The model under review builds one solid part; all positions refer to its coordinate system, in mm. Coordinates: 2 decimals unless noted, no trailing zeros. Loops run counter-clockwise (first coordinate to the right, second up) from the corner with the lowest first, then second, coordinate; pieces in that order, holes last. Notation, with made-up numbers: M -16,79 L 31,79 A8 cw 31,91 Z; hole C 34,-31 d7. An arc over 180 degrees is marked long. One line per item, written item: value.
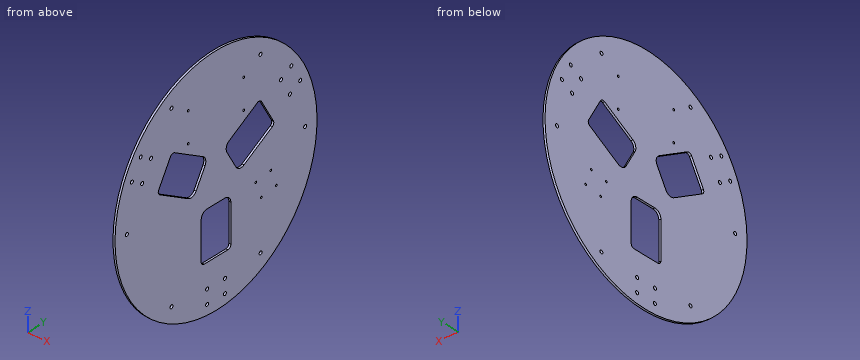
```python
from build123d import *

# Parameters (mm, degrees)
SKETCH_1_R      = 170
SKETCH_1_R_2    = 2.5
SKETCH_1_R_3    = 1.5
EXTRUDE_1_DEPTH = 3


with BuildPart() as part:
    # 草图1 → 凸台-拉伸1 (new body)
    with BuildSketch(Plane(origin=(0, 0, 0), x_dir=(0, 0, -1), z_dir=(1, 0, 0))):
        Circle(SKETCH_1_R)
        with Locations((155, 15)):
            Circle(SKETCH_1_R_2, mode=Mode.SUBTRACT)
        with Locations((135, 15)):
            Circle(SKETCH_1_R_2, mode=Mode.SUBTRACT)
        with Locations(Location((135, -15, 0), (0, 0, 180))):
            Circle(SKETCH_1_R_2, mode=Mode.SUBTRACT)
        with Locations(Location((155, -15, 0), (0, 0, 180))):
            Circle(SKETCH_1_R_2, mode=Mode.SUBTRACT)
        with Locations((-90.490381057, 126.733937587)):
            Circle(SKETCH_1_R_2, mode=Mode.SUBTRACT)
        with Locations((-80.490381057, 109.413429511)):
            Circle(SKETCH_1_R_2, mode=Mode.SUBTRACT)
        with Locations(Location((-54.509618943, 124.413429511, 0), (0, 0, 180))):
            Circle(SKETCH_1_R_2, mode=Mode.SUBTRACT)
        with Locations(Location((-64.509618943, 141.733937587, 0), (0, 0, 180))):
            Circle(SKETCH_1_R_2, mode=Mode.SUBTRACT)
        with Locations((-64.509618943, -141.733937587)):
            Circle(SKETCH_1_R_2, mode=Mode.SUBTRACT)
        with Locations((-54.509618943, -124.413429511)):
            Circle(SKETCH_1_R_2, mode=Mode.SUBTRACT)
        with Locations(Location((-80.490381057, -109.413429511, 0), (0, 0, 180))):
            Circle(SKETCH_1_R_2, mode=Mode.SUBTRACT)
        with Locations(Location((-90.490381057, -126.733937587, 0), (0, 0, 180))):
            Circle(SKETCH_1_R_2, mode=Mode.SUBTRACT)
        with Locations((-70, 46.6)):
            Circle(SKETCH_1_R_3, mode=Mode.SUBTRACT)
        with Locations((-113.2, 46.6)):
            Circle(SKETCH_1_R_3, mode=Mode.SUBTRACT)
        with Locations(Location((-113.2, -46.6, 0), (0, 0, 180))):
            Circle(SKETCH_1_R_3, mode=Mode.SUBTRACT)
        with Locations(Location((-70, -46.6, 0), (0, 0, 180))):
            Circle(SKETCH_1_R_3, mode=Mode.SUBTRACT)
        with Locations((0, -150)):
            Circle(SKETCH_1_R_2, mode=Mode.SUBTRACT)
        with Locations((-129.903810568, -75)):
            Circle(SKETCH_1_R_2, mode=Mode.SUBTRACT)
        with Locations((-129.903810568, 75)):
            Circle(SKETCH_1_R_2, mode=Mode.SUBTRACT)
        with Locations((0, 150)):
            Circle(SKETCH_1_R_2, mode=Mode.SUBTRACT)
        with Locations((129.903810568, 75)):
            Circle(SKETCH_1_R_2, mode=Mode.SUBTRACT)
        with Locations((129.903810568, -75)):
            Circle(SKETCH_1_R_2, mode=Mode.SUBTRACT)
        with Locations((54.035898385, 101.592921435)):
            Circle(SKETCH_1_R_3, mode=Mode.SUBTRACT)
        with Locations((34.035898385, 66.951905284)):
            Circle(SKETCH_1_R_3, mode=Mode.SUBTRACT)
        with Locations((57.892304845, 76.27241336)):
            Circle(SKETCH_1_R_3, mode=Mode.SUBTRACT)
        with Locations((30.179491924, 92.27241336)):
            Circle(SKETCH_1_R_3, mode=Mode.SUBTRACT)
        with BuildLine():
            Line((100, 0), (100, 20))
            ThreePointArc((100, 20), (98.535533906, 23.535533906), (95, 25))
            Line((95, 25), (40, 25))
            ThreePointArc((40, 25), (32.928932188, 22.071067812), (30, 15))
            Line((30, 15), (30, -15))
            ThreePointArc((30, -15), (32.928932188, -22.071067812), (40, -25))
            Line((40, -25), (95, -25))
            ThreePointArc((95, -25), (98.535533906, -23.535533906), (100, -20))
            Line((100, -20), (100, 0))
        make_face(mode=Mode.SUBTRACT)
        with BuildLine():
            Line((-50, 86.602540378), (-67.320508076, 76.602540378))
            ThreePointArc((-67.320508076, 76.602540378), (-69.650137207, 73.566508585), (-69.150635095, 69.77241336))
            Line((-69.150635095, 69.77241336), (-41.650635095, 22.141016151))
            ThreePointArc((-41.650635095, 22.141016151), (-35.578571508, 17.481757888), (-27.990381057, 18.480762114))
            Line((-27.990381057, 18.480762114), (-2.009618943, 33.480762114))
            ThreePointArc((-2.009618943, 33.480762114), (2.64963932, 39.5528257), (1.650635095, 47.141016151))
            Line((1.650635095, 47.141016151), (-25.849364905, 94.77241336))
            ThreePointArc((-25.849364905, 94.77241336), (-28.885396699, 97.102042491), (-32.679491924, 96.602540378))
            Line((-32.679491924, 96.602540378), (-50, 86.602540378))
        make_face(mode=Mode.SUBTRACT)
        with BuildLine():
            Line((-50, -86.602540378), (-32.679491924, -96.602540378))
            ThreePointArc((-32.679491924, -96.602540378), (-28.885396699, -97.102042491), (-25.849364905, -94.77241336))
            Line((-25.849364905, -94.77241336), (1.650635095, -47.141016151))
            ThreePointArc((1.650635095, -47.141016151), (2.64963932, -39.5528257), (-2.009618943, -33.480762114))
            Line((-2.009618943, -33.480762114), (-27.990381057, -18.480762114))
            ThreePointArc((-27.990381057, -18.480762114), (-35.578571508, -17.481757888), (-41.650635095, -22.141016151))
            Line((-41.650635095, -22.141016151), (-69.150635095, -69.77241336))
            ThreePointArc((-69.150635095, -69.77241336), (-69.650137207, -73.566508585), (-67.320508076, -76.602540378))
            Line((-67.320508076, -76.602540378), (-50, -86.602540378))
        make_face(mode=Mode.SUBTRACT)
    extrude(amount=EXTRUDE_1_DEPTH)


solid = part.part
```
(1) To check wall thickness, follow L1, parallel to Y at x = 1.9, z = 5; L2, parallel to Y at x = 1, z = 0; L3, parallel to Y at x = 2.45, z = 24.5. State the ranges of each line that lie inside material, in increasing order. Write a range as [from, to].
Checks:
L1: [-169.93, -58.66], [-31.75, 31.75], [58.66, 169.93]
L2: [-170, -152.5], [-147.5, -50], [-35.01, 35.01], [50, 147.5], [152.5, 170]
L3: [-168.23, -92.44], [-20.5, 20.5], [92.44, 168.23]
(2) Add section C-C on x = 0.7. State how many separate pieces and enclosed holes the cut face has, then the cut area to 3 significant figures.
Checks:
separate pieces: 1
enclosed holes: 29
area: 80,000 mm^2
(3) Add section A-A on y = -89. State the section outline as (x, z) points.
Checks:
outline: M 0,-144.84 L 3,-144.84 L 3,22.52 L 0,22.52 Z; M 0,45.85 L 3,45.85 L 3,144.84 L 0,144.84 Z
(4) Add section B-B on y = 4.5. State the section outline as (x, z) points, then the cut area to 3 significant figures.
Checks:
outline: M 0,-169.94 L 3,-169.94 L 3,-100 L 0,-100 Z; M 0,-30 L 3,-30 L 3,169.94 L 0,169.94 Z
area: 810 mm^2
(5) Insertion check: pin 1 Ø0.9 at (x, y) = (1.5, -4.5) entering from +Z. The pin has a flat end and moves straight along its axis. Give the tip position at first contact, or say it passes through.
Checks:
pin 1: z = 169.95
(6) Add section D-D on z = -121.5. State the section outline as (x, y) points.
Checks:
outline: M 0,-118.9 L 3,-118.9 L 3,118.9 L 0,118.9 Z
